```python
from build123d import *

# Parameters (mm, degrees)
SKETCH2_R      = 15
EXTRUDE1_DEPTH = 20


with BuildPart() as part:
    # Sketch1 → Revolve1 (revolve)
    with BuildSketch(Plane.XY, mode=Mode.PRIVATE) as revolve1_sk:
        Polygon((0, 21), (-98.5, 21), (-98.5, 19), (-137.5, 19), (-137.5, 16), (-150.5, 16), (-150.5, 15), (-170.5, 15), (-170.5, 12.5), (0, 12.5), align=None)
    revolve1 = revolve(revolve1_sk.sketch.rotate(Axis((0, 0, 0), (1, 0, 0)), 90), axis=Axis((0, 0, 0), (1, 0, 0)))

    # Mirror1: Revolve1 across plane
    add(revolve1.mirror(Plane(origin=(0, 0, 0), x_dir=(0, 0, 1), z_dir=(1, 0, 0))))

    # Sketch2 → Extrude1 (cut)
    with BuildSketch(Plane(origin=(170.5, 0, 0), x_dir=(0, 0, -1), z_dir=(1, 0, 0))):
        with Locations(Location((0, 0, 0), (0, 0, 180))):
            Circle(SKETCH2_R)
    extrude(amount=-EXTRUDE1_DEPTH, mode=Mode.SUBTRACT)


solid = part.part
```
Geometry check sheet. Reference: the model listing, model coordinates, mm. A direction names the side the tool comes from. Round coordinates to 2 decimals unless told otherwise and drop trailing zeros. Loops run counter-clockwise (first coordinate to the right, second up) from the corner with the lowest first, then second, coordinate; pieces in that order, holes last. Notation, with made-up numbers: (12, 55.25) -> (25, 55.25) arc R21 ccw to (25, 84.25) -> close; hole circle Ø8 at (16, 30). An arc over 180 degrees is marked (long way). Use a Markdown table: item, result.
(1) Scan lines: probe 1 along Y at (x, z) = (44.5, 0); probe 2 along X at (y, z) = (-5.5, 14.5); probe 3 along X at (y, z) = (-17.5, -4.5). Record each from-to range of solid material in increasing order.
Calculated:
| item | result |
|---|---|
| probe 1 | -21 to -12.5, 12.5 to 21 |
| probe 2 | -150.5 to 150.5 |
| probe 3 | -137.5 to 137.5 |
(2) Go/stop test with flat-tipped pins: P1, Ø1.5, axis at x = 25.5, y = -11.5, coming from the +Z side; P2, Ø3, axis at x = 77.5, z = -9, coming from the +Y side; P3, Ø5, axis at x = 95, y = -7, coming from the -Z side. Record where each tip stops, or that it passes through.
Calculated:
| item | result |
|---|---|
| P1 | z = 18.04 |
| P2 | y = 19.62 |
| P3 | z = -20.51 |
(3) Sectioned sample at D-D (x = -126.5). Enter the section's corners in (y, z).
Calculated:
| item | result |
|---|---|
| outline | circle Ø38 at (0, 0); hole circle Ø25 at (0, 0) |
(4) Set-up check for faces 1 (the flat face through (98.5, 11, -16)), 2 (the flat face through (-170.5, -12.3, -3.4)), 3 (the cylindrical face through (-118.273, 18.548, -4.119)): record each of +Z, -Z, +X, -X, +Y, -Y from which the full face is reachable in a straight line by a thin tool's end or side.
Calculated:
| item | result |
|---|---|
| face 1 | +X |
| face 2 | +Z, -Z, -X, +Y, -Y |
| face 3 | -X |
(5) Sectioned sample at C-C (x = -81). Enter the section's corners in (y, z), then the cut area to 3 significant figures.
Calculated:
| item | result |
|---|---|
| outline | circle Ø42 at (0, 0); hole circle Ø25 at (0, 0) |
| area | 895 mm² |
(6) Sectioned sample at A-A (z = 0). Enter the section's corners in (x, y), then the cut area to 4 significant figures.
Calculated:
| item | result |
|---|---|
| outline | (-170.5, -15) -> (-150.5, -15) -> (-150.5, -16) -> (-137.5, -16) -> (-137.5, -19) -> (-98.5, -19) -> (-98.5, -21) -> (98.5, -21) -> (98.5, -19) -> (137.5, -19) -> (137.5, -16) -> (150.5, -16) -> (150.5, -12.5) -> (-170.5, -12.5) -> close; (-170.5, 12.5) -> (150.5, 12.5) -> (150.5, 16) -> (137.5, 16) -> (137.5, 19) -> (98.5, 19) -> (98.5, 21) -> (-98.5, 21) -> (-98.5, 19) -> (-137.5, 19) -> (-137.5, 16) -> (-150.5, 16) -> (-150.5, 15) -> (-170.5, 15) -> close |
| area | 4,645 mm² |
